Build history of the part. All positions in model axes, mm. Face numbers are marked on the shaded views. A direction names the side the tool comes from. Coordinates: 2 decimals unless noted, no trailing zeros. Write each loop counter-clockwise with the first axis right and the second up, starting at its lowest first coordinate (ties: lowest second). Pieces come first, ordered by that corner, then holes. Notation, with made-up numbers: (87, 31.25) -> (101, 31.25) arc R22 cw to (101, 61.25) -> close; hole circle Ø5 at (79.25, 23.5). An arc over 180 degrees is marked (long way). Write each question's results on one line, items separated by ' | '. Start each with the question number.
Q1. Drill centre lines: line 1 (Y direction, x = 13.75, z = -2.75); line 2 (Z direction, x = -8.25, y = -15); line 3 (Y direction, x = -8.75, z = -4.5). Where is each one in solid material? Low to high.
Q2. Drop a flat-ended pin along its axis: pin 1 Ø1.5 at (x, y) = (6.5, 14) entering from -Z. Give the stop position or say it passes through.
Q3. Saw through at A-A on z = -2.5. Give the cut face in (x, y).
Q4. Saw through at C-C on y = 4. Give the cut face in (x, z).
Q5. Saw through at B-B on x = 5.25. Give the cut face in (y, z), and give its area (3 significant figures).
Q6. Tool access for the marked faces 1 and 2: list every direction of +Z, -Z, +X, -X, +Y, -Y with a clear straight run to the whole face (end or side of a thin tool).
from build123d import *

# Parameters (mm, degrees)
F0_W     = 25
F0_H     = 32.5
F0_W_2   = 2.5
F1_DEPTH = 5
F2_DEPTH = 5
F3_R     = 1


with BuildPart() as f1:
    # F0 (on Top) → F1 (new body)
    with BuildSketch(Plane.XY):
        Rectangle(F0_W, F0_H)
        Polygon((-15, 16.25), (-12.5, 16.25), (12.5, 16.25), (15, 16.25), (15, 18.75), (-15, 18.75), align=None)
        with Locations((-13.75, 0)):
            Rectangle(F0_W_2, F0_H)
        Polygon((12.5, -16.25), (-12.5, -16.25), (-15, -16.25), (-15, -18.75), (15, -18.75), (15, -16.25), align=None)
        with Locations((13.75, 0)):
            Rectangle(F0_W_2, F0_H)
    extrude(amount=F1_DEPTH)

    # F0 (on Top) → F2 (join)
    with BuildSketch(Plane.XY):
        Polygon((12.5, -16.25), (-12.5, -16.25), (-15, -16.25), (-15, -18.75), (15, -18.75), (15, -16.25), align=None)
        Polygon((-15, 16.25), (-12.5, 16.25), (12.5, 16.25), (15, 16.25), (15, 18.75), (-15, 18.75), align=None)
    extrude(amount=-F2_DEPTH)

    # F3
    f3_edges = [f1.edges().sort_by_distance(p)[0] for p in [
        (0, 16.25, -5),
        (15, 17.5, -5),
        (0, 18.75, -5),
        (-15, 17.5, -5),
        (-15, -17.5, -5),
        (0, -18.75, -5),
        (15, -17.5, -5),
        (0, -16.25, -5),
        (-15, 0, 5),
        (-15, -18.75, 0),
        (-15, -16.25, -2.5),
        (-15, 0, 0),
        (-15, 16.25, -2.5),
        (-15, 18.75, 0),
        (15, 18.75, 0),
        (0, 18.75, 5),
        (15, -18.75, 0),
        (15, 0, 5),
        (15, 16.25, -2.5),
        (15, 0, 0),
        (15, -16.25, -2.5),
        (0, -18.75, 5),
    ]]
    fillet(f3_edges, radius=F3_R)


solid = f1.part
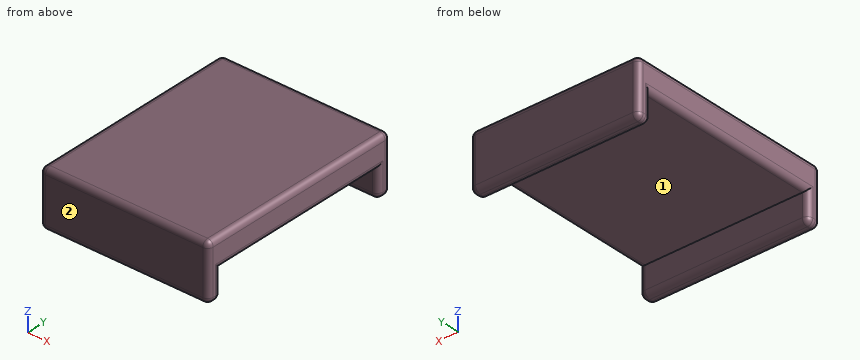
Returned:
1) line 1: y = -18.75 to -16.25, 16.25 to 18.75 | line 2: z = 0 to 5 | line 3: y = -18.62 to -16.38, 16.38 to 18.62
2) pin 1: stops at z = 0
3) outline: (-15, -17.75) arc R1 ccw to (-14, -18.75) -> (14, -18.75) arc R1 ccw to (15, -17.75) -> (15, -17.25) arc R1 ccw to (14, -16.25) -> (-14, -16.25) arc R1 ccw to (-15, -17.25) -> close; (-15, 17.25) arc R1 ccw to (-14, 16.25) -> (14, 16.25) arc R1 ccw to (15, 17.25) -> (15, 17.75) arc R1 ccw to (14, 18.75) -> (-14, 18.75) arc R1 ccw to (-15, 17.75) -> close
4) outline: (-15, 1) arc R1 ccw to (-14, 0) -> (14, 0) arc R1 ccw to (15, 1) -> (15, 4) arc R1 ccw to (14, 5) -> (-14, 5) arc R1 ccw to (-15, 4) -> close
5) outline: (-18.75, -4) arc R1 ccw to (-17.75, -5) -> (-17.25, -5) arc R1 ccw to (-16.25, -4) -> (-16.25, 0) -> (16.25, 0) -> (16.25, -4) arc R1 ccw to (17.25, -5) -> (17.75, -5) arc R1 ccw to (18.75, -4) -> (18.75, 4) arc R1 ccw to (17.75, 5) -> (-17.75, 5) arc R1 ccw to (-18.75, 4) -> close | area: 211 mm2
6) face 1: -Z, +X, -X | face 2: +Z, -Z, +X, -X, -Y
